```python
from build123d import *

# Parameters (mm, degrees)
SKETCH1_R           = 36.4744
BOSS_EXTRUDE1_DEPTH = 9.525
SKETCH2_R           = 26.543
BOSS_EXTRUDE2_DEPTH = 3.175
SKETCH5_R           = 3.175
SKETCH5_R_2         = 1.143
SKETCH5_R_3         = 4.191
SKETCH5_R_4         = 2.54
CUT_EXTRUDE1_DEPTH  = 54.123005475


with BuildPart() as part:
    # Sketch1 → Boss-Extrude1 (new body)
    with BuildSketch(Plane(origin=(0, 0, 0), x_dir=(1, 0, 0), z_dir=(0, 1, 0))):
        with Locations(Location((0, 0, 0), (0, 0, 270))):
            Circle(SKETCH1_R)
    extrude(amount=-BOSS_EXTRUDE1_DEPTH)

    # Sketch2 → Boss-Extrude2 (add)
    with BuildSketch(Plane.XZ.offset(9.525)):
        with Locations(Location((0, 0, 0), (0, 0, 270))):
            Circle(SKETCH2_R)
    extrude(amount=BOSS_EXTRUDE2_DEPTH)

    # Sketch5 → Cut-Extrude1 (cut, through all)
    with BuildSketch(Plane(origin=(0, 0, 0), x_dir=(1, 0, 0), z_dir=(0, 1, 0))):
        with Locations(Location((0, 0, 0), (0, 0, 270))):
            Circle(SKETCH5_R)
        with Locations(Location((-6.279225326, 19.325468411, 0), (0, 0, 270))):
            Circle(SKETCH5_R_2)
        with Locations(Location((-20.533310187, -6.671676909, 0), (0, 0, 270))):
            Circle(SKETCH5_R_3)
        with Locations(Location((-15.266435406, -15.266435406, 0), (0, 0, 270))):
            Circle(SKETCH5_R)
        with Locations(Location((15.266435406, 15.266435406, 0), (0, 0, 270))):
            Circle(SKETCH5_R)
        with Locations(Location((6.279225326, -19.325468411, 0), (0, 0, 270))):
            Circle(SKETCH5_R_2)
        with Locations(Location((20.533310187, 6.671676909, 0), (0, 0, 270))):
            Circle(SKETCH5_R_3)
        with Locations(Location((21.293906137, -3.563377811, 0), (0, 0, 270))):
            Circle(SKETCH5_R_4)
        with Locations(Location((-21.293906137, 3.563377811, 0), (0, 0, 270))):
            Circle(SKETCH5_R_4)
    extrude(amount=-CUT_EXTRUDE1_DEPTH, mode=Mode.SUBTRACT)


solid = part.part
```
The model under review builds one solid part; all positions refer to its coordinate system, in mm. Coordinates: 2 decimals unless noted, no trailing zeros. Write each loop counter-clockwise with the first axis right and the second up, starting at its lowest first coordinate (ties: lowest second). Pieces come first, ordered by that corner, then holes.
1) We need section A-A on z = 0. State the section outline as (x, y) points (3 decimals), then the cut area to 3 significant figures.
2) Clearance check with flat-ended pins moving along their axes: pin 1 Ø1.5 at (x, y) = (25.5, -6.5) entering from -Z; pin 2 Ø5 at (y, z) = (-6.5, 25.5) entering from -X; pin 3 Ø6 at (x, y) = (19, -8.5) entering from +Z. State where each tip first meets the part, or that it passes through.
3) We need section D-D on x = 23. State the section outline as (y, z) points (3 decimals).
4) To check wall thickness, follow probe 1 along X at (y, z) = (-4, 0) (3 decimals); probe 2 along Z at (x, y) = (-21, -6.75); probe 3 along X at (y, z) = (-10.5, -1.5). State the ranges of each line that lie inside material, in increasing order.
5) We need section C-C on y = -3. Count the separate pieces of the cut face and the enclosed holes in it, then the cut area to 3 significant figures.
6) We need section B-B on x = 0. State the section outline as (y, z) points (3 decimals).
7) The part is to be moulded in two halves that separate along Z. For faces 1 (the face through (-27, -9.525, 3)), 2 (the face through (-22.84, -6.26, -5.58)), 3 (the face through (-25.9, -11.1, 5.8)), say which applies: pulls with the +Z half, pulls with the -Z half, needs draft (parallel to the pull), parting line crosses it, or undercut.
Answer list:
1. outline: (-36.474, -9.525) - (-26.543, -9.525) - (-26.543, -12.7) - (-3.175, -12.7) - (-3.175, 0) - (-36.474, 0) - close; (3.175, -12.7) - (26.543, -12.7) - (26.543, -9.525) - (36.474, -9.525) - (36.474, 0) - (3.175, 0) - close
1. area: 783 mm2
2. pin 1: stops at z = -26.79
2. pin 2: stops at x = -28.31
2. pin 3: stops at z = 32.78
3. outline: (-12.7, -13.249) - (-9.525, -13.249) - (-9.525, -28.309) - (0, -28.309) - (0, -10.06) - (-12.7, -10.06) - close; (-12.7, -3.283) - (0, -3.283) - (0, 1.682) - (-12.7, 1.682) - close; (-12.7, 5.445) - (0, 5.445) - (0, 28.309) - (-9.525, 28.309) - (-9.525, 13.249) - (-12.7, 13.249) - close
4. probe 1: x = -36.474 to -3.175, 3.175 to 36.474
4. probe 2: z = -29.82 to -6.09, -1.04 to 2.51, 10.84 to 29.82
4. probe 3: x = -26.5 to -22.78, -19.81 to -2.8, 2.8 to 26.5
5. separate pieces: 1
5. enclosed holes: 9
5. area: 3,930 mm2
6. outline: (-12.7, -26.543) - (-9.525, -26.543) - (-9.525, -36.474) - (0, -36.474) - (0, -3.175) - (-12.7, -3.175) - close; (-12.7, 3.175) - (0, 3.175) - (0, 36.474) - (-9.525, 36.474) - (-9.525, 26.543) - (-12.7, 26.543) - close
7. face 1: needs draft
7. face 2: undercut
7. face 3: parting line crosses it
